Could you check a few things on this model? Use its own coordinates, in mm. Face numbers are marked on the shaded views. A direction names the side the tool comes from. Round coordinates to 2 decimals unless told otherwise and drop trailing zeros. Order: outer loops, then holes, each group sorted by start corner. A loop starts at its lowest first (then second) coordinate and runs counter-clockwise, first axis right, second up.
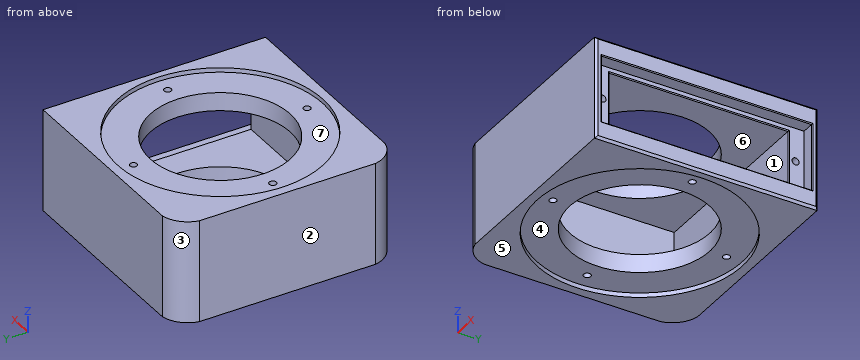
```python
from build123d import *

# Parameters (mm, degrees)
SKETCH005_W     = 50
SKETCH005_H     = 50
SKETCH005_R     = 15.69193
PAD_DEPTH       = 23
SKETCH006_W     = 40.8
SKETCH006_H     = 12.8
POCKET_DEPTH    = 40.2
SKETCH011_W     = 47.2
SKETCH011_H     = 15
POCKET001_DEPTH = 3
SKETCH012_R     = 0.8
SKETCH012_W     = 40.2
SKETCH012_H     = 12.8
POCKET002_DEPTH = 5
SKETCH020_R     = 23
POCKET007_DEPTH = 1
SKETCH021_R     = 23
POCKET008_DEPTH = 1
SKETCH022_R     = 0.8
POCKET009_DEPTH = 5
SKETCH023_R     = 0.8
POCKET010_DEPTH = 5
POCKET015_DEPTH = 23.001
CHAMFER012_SIZE = 0.2
CHAMFER_SIZE    = 0.5


with BuildPart() as part:
    # Sketch005 → Pad (new body)
    with BuildSketch(Plane.XY):
        Rectangle(SKETCH005_W, SKETCH005_H)
        Circle(SKETCH005_R, mode=Mode.SUBTRACT)
    extrude(amount=PAD_DEPTH)

    # Sketch006 → Pocket (cut)
    with BuildSketch(Plane.XZ.offset(20.1)):
        with Locations((0, 11.5)):
            Rectangle(SKETCH006_W, SKETCH006_H)
    extrude(amount=-POCKET_DEPTH, mode=Mode.SUBTRACT)

    # Sketch011 → Pocket001 (cut)
    with BuildSketch(Plane.YZ.offset(25)):
        with Locations((0, 11.5)):
            Rectangle(SKETCH011_W, SKETCH011_H)
    extrude(amount=-POCKET001_DEPTH, mode=Mode.SUBTRACT)

    # Sketch012 → Pocket002 (cut)
    with BuildSketch(Plane.YZ.offset(22)):
        with Locations((-21.7, 11.5)):
            Circle(SKETCH012_R)
        with Locations((21.7, 11.5)):
            Circle(SKETCH012_R)
        with Locations((0, 11.5)):
            Rectangle(SKETCH012_W, SKETCH012_H)
    extrude(amount=-POCKET002_DEPTH, mode=Mode.SUBTRACT)

    # Sketch020 → Pocket007 (cut)
    with BuildSketch(Plane.XY):
        Circle(SKETCH020_R)
    extrude(amount=POCKET007_DEPTH, mode=Mode.SUBTRACT)

    # Sketch021 → Pocket008 (cut)
    with BuildSketch(Plane.XY.offset(23.01)):
        Circle(SKETCH021_R)
    extrude(amount=-POCKET008_DEPTH, mode=Mode.SUBTRACT)

    # Sketch022 → Pocket009 (cut)
    with BuildSketch(Plane.XY):
        with Locations((-19.5, 0)):
            Circle(SKETCH022_R)
        with Locations((0, -19.5)):
            Circle(SKETCH022_R)
        with Locations((19.5, 0)):
            Circle(SKETCH022_R)
        with Locations((0, 19.5)):
            Circle(SKETCH022_R)
    extrude(amount=POCKET009_DEPTH, mode=Mode.SUBTRACT)

    # Sketch023 → Pocket010 (cut)
    with BuildSketch(Plane.XY.offset(23)):
        with Locations((-19.5, 0)):
            Circle(SKETCH023_R)
        with Locations((0, -19.5)):
            Circle(SKETCH023_R)
        with Locations((19.5, 0)):
            Circle(SKETCH023_R)
        with Locations((0, 19.5)):
            Circle(SKETCH023_R)
    extrude(amount=-POCKET010_DEPTH, mode=Mode.SUBTRACT)

    # Sketch033 → Pocket015 (cut, through all)
    with BuildSketch(Plane.XY):
        with BuildLine():
            Line((-19, 25.1), (-25.1, 25.1))
            Line((-25.1, 19), (-25.1, 25.1))
            ThreePointArc((-19, 25.1), (-23.203288, 23.203288), (-25.1, 19))
        make_face()
        with BuildLine():
            Line((-25.1, -19), (-25.1, -25.1))
            Line((-19, -25.1), (-25.1, -25.1))
            ThreePointArc((-25.1, -19), (-23.203288, -23.203288), (-19, -25.1))
        make_face()
    extrude(amount=POCKET015_DEPTH, mode=Mode.SUBTRACT)

    # Chamfer012
    chamfer012_edges = [part.edges().sort_by_distance(p)[0] for p in [
        (22, 0, 5.1),
        (22, 20.1, 11.5),
        (22, 0, 17.9),
        (22, -20.1, 11.5),
        (25, -23.6, 11.5),
        (25, 0, 4),
        (25, 23.6, 11.5),
        (25, 0, 19),
    ]]
    chamfer(chamfer012_edges, length=CHAMFER012_SIZE)

    # Chamfer
    chamfer_edges = [part.edges().sort_by_distance(p)[0] for p in [
        (25, 25, 11.5),
        (25, 0, 0),
        (25, 0, 23),
        (25, -25, 11.5),
    ]]
    chamfer(chamfer_edges, length=CHAMFER_SIZE)


with BuildPart() as part_1:
    # Body002 placement: moved
    add(part.part.moved(Location((0, 0, -2))))


solid = part_1.part
```
Q1. I need wall thicknesses on L1, parallel to X at y = 0, z = -0.05; L2, parallel to Y at x = 10, z = 3.5. Which ranges of each line are inside material? Lowest first, please.
Q2. We'd pull the mould along Y, two halves only. Please class the marked faces 1, 2 and 3: released by +Y, released by -Y, zero draft, split by the parting line, or undercut.
Q3. For the marked faces 4, 5, 6 and 7, which set-ups out of +Z, -Z, +X, -X, +Y, -Y let a thin tool reach every point of the face, with its end or its side?
Q4. For P1, Ø10, axis at x = -6.5, y = 12.5, coming from the +Z side; P2, Ø1, axis at x = 0, y = 19.5, coming from the -Z side; P3, Ø1, axis at y = -18.5, z = 3.5, coming from the +X side; P4, Ø5, axis at x = 4.5, y = -12, coming from the +Z side, each with a flat end and sliding along its axis, tell me the tip position at first contact or that it passes through.
Q5. Imagine slicing it at A-A, the plane y = -7. State how many separate pieces and enclosed holes the cut face has, then the cut area to 3 significant figures.
Q6. Imagine slicing it at D-D, the plane z = 19. Please give me the cut outline in (x, y), then the cut area to 3 significant figures.
Q7. Imagine slicing it at C-C, the plane x = -13.5. Please give me the cut outline in (y, z), then the cut area to 3 significant figures.
Q8. Imagine slicing it at B-B, the plane z = 3.75. Please give me the cut outline in (x, y).
Filled in:
1. L1: x = -25 to -20.3, -18.7 to -15.69, 15.69 to 18.7, 20.3 to 25
1. L2: y = -25 to -20.1, 20.1 to 25
2. face 1: undercut
2. face 2: zero draft
2. face 3: released by +Y
3. face 4: -Z
3. face 5: -Z, +X, -X, +Y, -Y
3. face 6: +X
3. face 7: +Z
4. P1: stops at z = 20.01
4. P2: stops at z = 3
4. P3: stops at x = 21.9
4. P4: passes through
5. separate pieces: 3
5. enclosed holes: 0
5. area: 244 mm2
6. outline: (-25, -19.8) arc R6.52 ccw to (-19.8, -25) - (24.5, -25) - (25, -24.5) - (25, 24.5) - (24.5, 25) - (-19.8, 25) arc R6.52 ccw to (-25, 19.8) - close; hole circle Ø1.6 at (-19.5, 0); hole circle Ø31.38 at (0, 0); hole circle Ø1.6 at (0, -19.5); hole circle Ø1.6 at (0, 19.5); hole circle Ø1.6 at (19.5, 0)
6. area: 1,700 mm2
7. outline: (-25, -2) - (-18.62, -2) - (-18.62, -1) - (-8, -1) - (-8, 3.1) - (-20.1, 3.1) - (-20.1, 15.9) - (-8, 15.9) - (-8, 20.01) - (-18.62, 20.01) - (-18.62, 21) - (-25, 21) - close; (8, -1) - (18.62, -1) - (18.62, -2) - (25, -2) - (25, 21) - (18.62, 21) - (18.62, 20.01) - (8, 20.01) - (8, 15.9) - (20.1, 15.9) - (20.1, 3.1) - (8, 3.1) - close
7. area: 430 mm2
8. outline: (-25, -19.8) arc R6.52 ccw to (-19.8, -25) - (24.5, -25) - (25, -24.5) - (25, -23.8) - (24.8, -23.6) - (22, -23.6) - (22, -20.3) - (21.8, -20.1) - (-20.4, -20.1) - (-20.4, 20.1) - (21.8, 20.1) - (22, 20.3) - (22, 23.6) - (24.8, 23.6) - (25, 23.8) - (25, 24.5) - (24.5, 25) - (-19.8, 25) arc R6.52 ccw to (-25, 19.8) - close
